from build123d import *

# Parameters (mm, degrees)
F0_W     = 50.8
F0_H     = 50.8
F0_W_2   = 47.625
F0_H_2   = 47.625
F1_DEPTH = 635
F2_R     = 1.5875
F3_R     = 1.5875


with BuildPart() as f1:
    # F0 (on Top) → F1 (new body)
    with BuildSketch(Plane.XY):
        with Locations((-12.7, -11.264074)):
            Rectangle(F0_W, F0_H)
        with Locations((-12.7, -11.264074)):
            Rectangle(F0_W_2, F0_H_2, mode=Mode.SUBTRACT)
    extrude(amount=-F1_DEPTH)

    # F2
    f2_edges = [f1.edges().sort_by_distance(p)[0] for p in [
        (-38.1, -36.664074, -317.5),
        (12.7, -36.664074, -317.5),
        (12.7, 14.135926, -317.5),
        (-38.1, 14.135926, -317.5),
    ]]
    fillet(f2_edges, radius=F2_R)

    # F3
    f3_edges = [f1.edges().sort_by_distance(p)[0] for p in [
        (-36.5125, 12.548426, -317.5),
        (11.1125, 12.548426, -317.5),
        (11.1125, -35.076574, -317.5),
        (-36.5125, -35.076574, -317.5),
    ]]
    fillet(f3_edges, radius=F3_R)


solid = f1.part
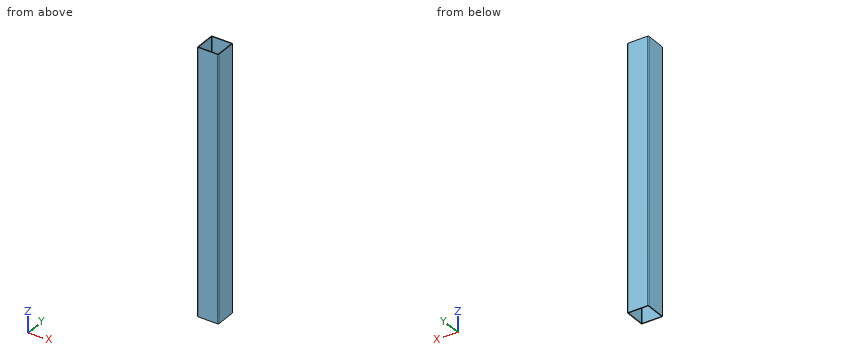
The model under review builds one solid part; all positions refer to its coordinate system, in mm. Round coordinates to 2 decimals unless told otherwise and drop trailing zeros. Loops run counter-clockwise (first coordinate to the right, second up) from the corner with the lowest first, then second, coordinate; pieces in that order, holes last. Notation, with made-up numbers: (28.25, 50) - (38.25, 50) arc R14 cw to (38.25, 54) - close; hole circle Ø11 at (71, -33). An arc over 180 degrees is marked (long way). Use CSV: the item, a comma, the result in double quotes.
(1) Take a section at C-C, the plane z = -370. Give the boundary of the cut face in (x, y) (1 decimal).
Working result:
outline,"(-38.1, -35.1) arc R1.6 ccw to (-36.5, -36.7) - (11.1, -36.7) arc R1.6 ccw to (12.7, -35.1) - (12.7, 12.5) arc R1.6 ccw to (11.1, 14.1) - (-36.5, 14.1) arc R1.6 ccw to (-38.1, 12.5) - close; hole (-36.5, -33.5) arc R1.6 ccw to (-34.9, -35.1) - (9.5, -35.1) arc R1.6 ccw to (11.1, -33.5) - (11.1, 11) arc R1.6 ccw to (9.5, 12.5) - (-34.9, 12.5) arc R1.6 ccw to (-36.5, 11) - close"
(2) Clearance check with a flat-ended pin moving along its axis: P1, Ø12, axis at x = -30, y = -6.5, coming from the -Z side. State where the tip first meets the part, or that it passes through.
Working result:
P1,"passes through"
(3) Take a section at A-A, the plane y = -18. Give the boundary of the cut face in (x, z).
Working result:
outline,"(-38.1, -635) - (-36.51, -635) - (-36.51, 0) - (-38.1, 0) - close; (11.11, -635) - (12.7, -635) - (12.7, 0) - (11.11, 0) - close"
(4) For line 1 (Y direction, x = 7.5, z = -138.5); line 2 (X direction, y = -30.5, z = -428), list the stretches that pass through material, from the lowest coordinate up.
Working result:
line 1,"y = -36.66 to -35.08, 12.55 to 14.14"
line 2,"x = -38.1 to -36.51, 11.11 to 12.7"
(5) Take a section at B-B, the plane x = -29.5. Give the boundary of the cut face in (y, z), plus the area to 3 significant figures.
Working result:
outline,"(-36.66, -635) - (-35.08, -635) - (-35.08, 0) - (-36.66, 0) - close; (12.55, -635) - (14.14, -635) - (14.14, 0) - (12.55, 0) - close"
area,"2,020 mm^2"
